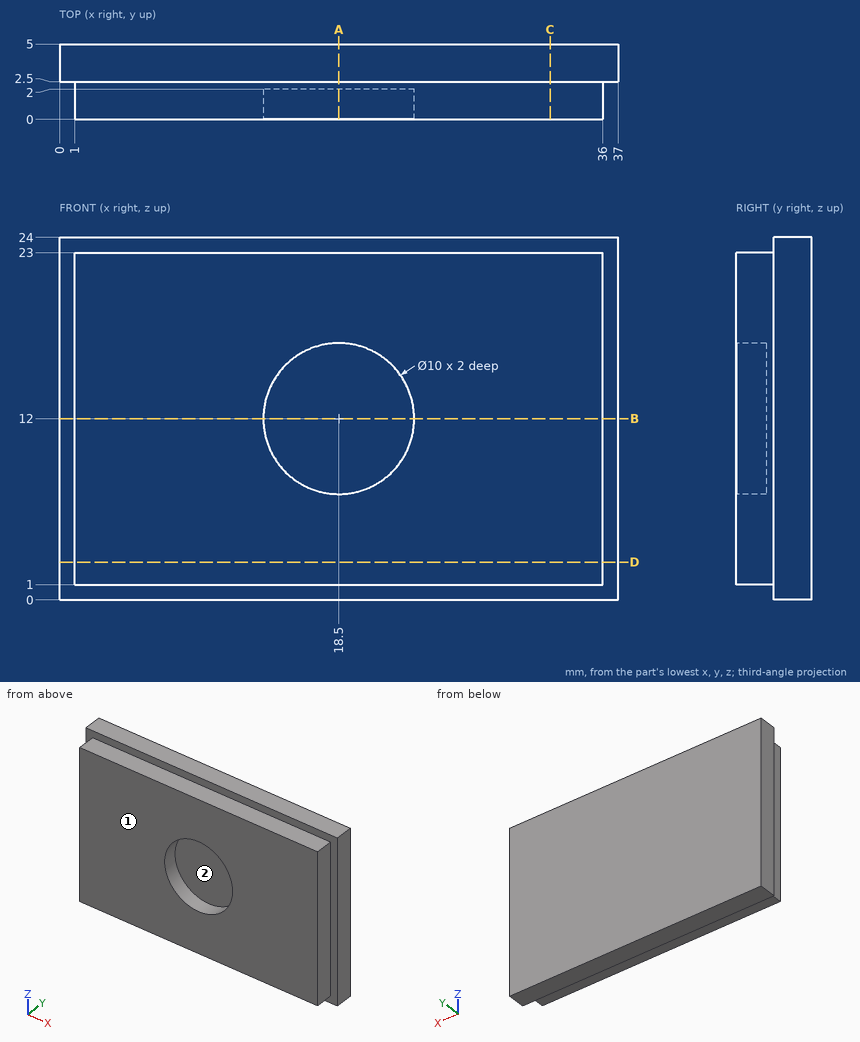
Answer from the drawing. Dimensions are ordinates in mm from the lowest x, y and z of the part. Give positions to 0.01 mm unless a question says otherwise; leave off trailing zeros. Write each loop counter-clockwise with the first axis right and the second up, starting at its lowest first coordinate (ties: lowest second). Pieces come first, ordered by that corner, then holes.
1) For a pull along Z with two mould halves and no side action, classify the marked faces 1 and 2 as pulls with the +Z half, pulls with the -Z half, needs draft (parallel to the pull), parting line crosses it, or undercut.
2) Section D-D (z = 2.5) is taken. Write down the section's boundary in (x, y), and give its area (3 significant figures).
3) Section C-C (x = 32.5) is taken. Write down the section's boundary in (y, z), and give its area (3 significant figures).
4) Section A-A (x = 18.5) is taken. Write down the section's boundary in (y, z).
5) Section B-B (z = 12) is taken. Write down the section's boundary in (x, y).
6) Given P1, Ø1.2, axis at x = 18.5, y = 0.5, coming from the -Z side; P2, Ø2, axis at x = 11.5, y = 1, coming from the +Z side; P3, Ø2, axis at y = 1, z = 14.5, coming from the +X side, each flat-ended and moving along its own axis, determine where each tip first touches the part or whether it passes through.
7) Find the intervals of material crossed by L1, parallel to Z at x = 18.5, y = 1.1; L2, parallel to Y at x = 20.5, z = 7.5; L3, parallel to X at y = 0.85, z = 14.5, in increasing order.
Response:
1. face 1: needs draft
1. face 2: undercut
2. outline: (0, 2.5) - (1, 2.5) - (1, 0) - (36, 0) - (36, 2.5) - (37, 2.5) - (37, 5) - (0, 5) - close
2. area: 180 mm2
3. outline: (0, 1) - (2.5, 1) - (2.5, 0) - (5, 0) - (5, 24) - (2.5, 24) - (2.5, 23) - (0, 23) - close
3. area: 115 mm2
4. outline: (0, 1) - (2.5, 1) - (2.5, 0) - (5, 0) - (5, 24) - (2.5, 24) - (2.5, 23) - (0, 23) - (0, 17) - (2, 17) - (2, 7) - (0, 7) - close
5. outline: (0, 2.5) - (1, 2.5) - (1, 0) - (13.5, 0) - (13.5, 2) - (23.5, 2) - (23.5, 0) - (36, 0) - (36, 2.5) - (37, 2.5) - (37, 5) - (0, 5) - close
6. P1: stops at z = 1
6. P2: stops at z = 23
6. P3: stops at x = 36
7. L1: z = 1 to 7, 17 to 23
7. L2: y = 2 to 5
7. L3: x = 1 to 14.17, 22.83 to 36
